from build123d import *

# Parameters (mm, degrees)
REDONDEO1_R                      = 0.762
TALADRO_DE_MARGEN_PARA_101_D     = 2.3622
TALADRO_DE_MARGEN_PARA_101_DEPTH = 0.8636
TALADRO_DE_MARGEN_PARA_101_TIP   = 0.709676477
CHAFL_N1_SIZE2                   = 0.337288027
CHAFL_N1_SIZE                    = 0.5842


# Some blends are built 0.0001 mm under size
with BuildPart() as part:
    # Croquis1 → Revolución1 (revolve)
    with BuildSketch(Plane(origin=(0, 0, 0), x_dir=(0, 0, -1), z_dir=(1, 0, 0)), mode=Mode.PRIVATE) as revoluci_n1_sk:
        Polygon((-13.4874, 0), (-13.4874, 1.9812), (-2.9464, 1.9812), (-2.9464, 1.8542), (-2.8194, 1.8542), (-2.8194, 1.9812), (-1.397, 1.9812), (-1.397, 1.8542), (-1.27, 1.8542), (-1.27, 1.9812), (0.1524, 1.9812), (0.1524, 1.8542), (0.2794, 1.8542), (0.2794, 1.9812), (3.3274, 1.9812), (3.3274, 1.7653), (13.4874, 1.7653), (13.4874, 0), align=None)
    revolve(revoluci_n1_sk.sketch.rotate(Axis((0, 0, 127), (0, 0, -1)), 90), axis=Axis((0, 0, 127), (0, 0, -1)))

    # Redondeo1
    # the kernel refuses this fillet: 0.762 mm, written as the material it adds along each edge
    with BuildSketch(Plane(origin=(0, 0, -3.3274), x_dir=(1, 0, 0), z_dir=(0, 1, 0))) as redondeo1_piece_1:
        with BuildLine():
            CenterArc((2.5273, 0.531430889), REDONDEO1_R, 180, 44.220044428)
            Line((1.7653, 0.531430889), (1.75006, 0.531430889))
            Line((1.75006, 0.531430889), (1.75006, 0))
            Line((1.75006, 0), (1.7653, -0.01524))
            ThreePointArc((1.7653, -0.01524), (1.87325, -0.01524), (1.970278, -0.010628618))
            Line((1.970278, -0.010628618), (1.9812, 0))
        make_face()
    revolve(axis=Axis((0, 0, -3.3274), (0, 0, -1)))

    # Taladro de margen para #101
    with Locations(Plane(origin=(0, 0, -13.4874), x_dir=(-1, 0, 0), z_dir=(0, 0, -1))):
        with Locations((0, 0)):
            Hole(TALADRO_DE_MARGEN_PARA_101_D / 2, depth=TALADRO_DE_MARGEN_PARA_101_DEPTH)
            with Locations((0, 0, -(TALADRO_DE_MARGEN_PARA_101_DEPTH + TALADRO_DE_MARGEN_PARA_101_TIP / 2))):  # 118° drill point
                Cone(0, TALADRO_DE_MARGEN_PARA_101_D / 2, TALADRO_DE_MARGEN_PARA_101_TIP, mode=Mode.SUBTRACT)

    # Chaflán1
    chafl_n1_edges = [part.edges().sort_by_distance(p)[0] for p in [
        (-1.1811, 0, -13.4874),
    ]]
    chafl_n1_side = [part.faces().sort_by_distance(p)[0] for p in [
        (-1.187845761, 0, -13.4874),
    ]]
    chamfer(chafl_n1_edges, length=CHAFL_N1_SIZE - 0.0001, length2=CHAFL_N1_SIZE2 - 0.0001, reference=chafl_n1_side[0])  # a hair under: the kernel refuses the full size


solid = part.part
The model under review builds one solid part; all positions refer to its coordinate system, in mm. A direction names the side the tool comes from. Coordinates: 2 decimals unless noted, no trailing zeros. Write each loop counter-clockwise with the first axis right and the second up, starting at its lowest first coordinate (ties: lowest second). Pieces come first, ordered by that corner, then holes. Notation, with made-up numbers: (-31.75, 69.5) - (1.25, 69.5) arc R17 cw to (1.25, 88.5) - close; hole circle Ø10 at (36.5, 38). An arc over 180 degrees is marked (long way). Answer as a JSON object with one key per item and string values. Group by question number.
1. Clearance check with flat-ended pins moving along their axes: pin 1 Ø2 at (x, y) = (0, 0.5) entering from -Z; pin 2 Ø1.5 at (y, z) = (-1.5, 6) entering from +X; pin 3 Ø1.2 at (x, y) = (-0.5, -1) entering from -Z. State where each tip first meets the part, or that it passes through.
2. Machinability: for faces 1 (the face through (-0.383, 1.723, -8.741)), 2 (the face through (-1.46, -1.34, -1.82)), which of the approach directions +Z, -Z, +X, -X, +Y, -Y give a long, thin tool a straight path to every point of the face, cutting with its end or side? Answer none if there is none.
3. To check wall thickness, follow probe 1 along X at (y, z) = (0, -12.8); probe 2 along Y at (x, z) = (-0.7, 1.5). State the ranges of each line that lie inside material, in increasing order.
4. Add section B-B (z = -6.5). Give the boundary of the cut face in (x, y).
5. Mouldability with a two-part tool opening along X and no side actions: class faces 3 (the face through (0, 0, 13.487)), 4 (the face through (-1.46, -1.34, 2.1)), 5 (the face through (0.63, 1, -12.88)) as pulls with the +X half, pulls with the -X half, needs draft (parallel to the pull), parting line crosses it, or undercut.
6. Add section A-A (z = 5.25). Give the boundary of the cut face in (x, y).
Findings:
{
 "1": {"pin 1": "z = -13.33", "pin 2": "x = 1.83", "pin 3": "z = -13.46"},
 "2": {"face 1": "-Z", "face 2": "+Z, -Z"},
 "3": {"probe 1": "-1.77 to -1.18, 1.18 to 1.77", "probe 2": "-1.85 to 1.85"},
 "4": {"outline": "circle Ø3.53 at (0, 0)"},
 "5": {"face 3": "needs draft", "face 4": "parting line crosses it", "face 5": "undercut"},
 "6": {"outline": "circle Ø3.96 at (0, 0)"}
}
